from build123d import *

# Parameters (mm, degrees)
SKETCH_1_R      = 33.5
SKETCH_1_R_2    = 23.5
EXTRUDE_1_DEPTH = 25
SKETCH_2_R      = 10
EXTRUDE_2_DEPTH = 2
SKETCH_3_R      = 5
SKETCH_3_R_2    = 2.5
EXTRUDE_3_DEPTH = 20


with BuildPart() as part:
    # 草圖1 → 填料-伸長1 (new body)
    with BuildSketch(Plane.XY):
        Circle(SKETCH_1_R)
        Circle(SKETCH_1_R_2, mode=Mode.SUBTRACT)
    extrude(amount=EXTRUDE_1_DEPTH)

    # 草圖2 → 填料-伸長2 (add)
    with BuildSketch(Plane(origin=(0, 0, 0), x_dir=(-1, 0, 0), z_dir=(0, 0, -1))):
        with BuildLine():
            ThreePointArc((-5, 8.660254038), (-2.588190451, 9.659258263), (0, 10))
            Line((0, 10), (0, 23.5))
            ThreePointArc((0, 23.5), (-1.251777149, 23.46663704), (-2.5, 23.366642891))
            Line((-2.5, 23.366642891), (-5, 8.660254038))
        make_face()
        with BuildLine():
            Line((0, 23.5), (0, 10))
            ThreePointArc((0, 10), (2.588190451, 9.659258263), (5, 8.660254038))
            Line((5, 8.660254038), (2.5, 23.366642891))
            ThreePointArc((2.5, 23.366642891), (1.251777149, 23.46663704), (0, 23.5))
        make_face()
        Circle(SKETCH_2_R)
        with BuildLine():
            ThreePointArc((-9.781476007, -2.079116908), (-9.510565163, 3.090169944), (-6.691306064, 7.431448255))
            Line((-6.691306064, 7.431448255), (-21.4504555, 9.598331046))
            ThreePointArc((-21.4504555, 9.598331046), (-22.349828133, 7.261899368), (-22.995540471, 4.843048464))
            Line((-22.995540471, 4.843048464), (-9.781476007, -2.079116908))
        make_face()
        with BuildLine():
            ThreePointArc((-1.045284633, -9.945218954), (-5.877852523, -8.090169944), (-9.135454576, -4.067366431))
            Line((-9.135454576, -4.067366431), (-15.757110573, -17.43454807))
            ThreePointArc((-15.757110573, -17.43454807), (-13.812953429, -19.011899368), (-11.712025601, -20.373474331))
            Line((-11.712025601, -20.373474331), (-1.045284633, -9.945218954))
        make_face()
        with BuildLine():
            Line((15.757110573, -17.43454807), (9.135454576, -4.067366431))
            ThreePointArc((9.135454576, -4.067366431), (5.877852523, -8.090169944), (1.045284633, -9.945218954))
            Line((1.045284633, -9.945218954), (11.712025601, -20.373474331))
            ThreePointArc((11.712025601, -20.373474331), (13.812953429, -19.011899368), (15.757110573, -17.43454807))
        make_face()
        with BuildLine():
            Line((21.4504555, 9.598331046), (6.691306064, 7.431448255))
            ThreePointArc((6.691306064, 7.431448255), (9.135454576, 4.067366431), (10, 0))
            ThreePointArc((10, 0), (9.945218954, -1.045284633), (9.781476007, -2.079116908))
            Line((9.781476007, -2.079116908), (22.995540471, 4.843048464))
            ThreePointArc((22.995540471, 4.843048464), (22.349828133, 7.261899368), (21.4504555, 9.598331046))
        make_face()
    extrude(amount=-EXTRUDE_2_DEPTH)

    # 草圖3 → 填料-伸長3 (add)
    with BuildSketch(Plane.XY.offset(2)):
        with Locations(Location((0, 0, 0), (0, 0, 180))):
            Circle(SKETCH_3_R)
        Circle(SKETCH_3_R_2, mode=Mode.SUBTRACT)
    extrude(amount=EXTRUDE_3_DEPTH)


solid = part.part
Work out the finished part from the listing and answer in its coordinate system (mm). A direction names the side the tool comes from. Give positions to 0.01 mm unless a question says otherwise; leave off trailing zeros. Loops run counter-clockwise (first coordinate to the right, second up) from the corner with the lowest first, then second, coordinate; pieces in that order, holes last. Notation, with made-up numbers: (50, 29.5) - (96, 29.5) arc R15 ccw to (96, 56.5) - close; hole circle Ø6 at (12, 60.25). An arc over 180 degrees is marked (long way). Answer in a Markdown table with one row per item.
(1) Flat-ended cylindrical pins translate along their axes: pin 1 Ø4 at (y, z) = (-8, 22) entering from -X; pin 2 Ø3 at (x, y) = (0, 0) entering from -Z; pin 3 Ø3 at (y, z) = (-23, 5) entering from -X; pin 4 Ø3 at (x, y) = (-1.5, -1.5) entering from +Z. Find the tip coordinate at first contact, or state that the pin passes through.
Results list:
| item | result |
|---|---|
| pin 1 | stops at x = -32.96 |
| pin 2 | stops at z = 0 |
| pin 3 | stops at x = -25.69 |
| pin 4 | stops at z = 22 |
(2) Section D-D (x = -17.5) is taken. Give the vertices of the cut face in (y, z).
Results list:
| item | result |
|---|---|
| outline | (-28.57, 0) - (-15.68, 0) - (-15.68, 25) - (-28.57, 25) - close; (1.96, 0) - (9.02, 0) - (9.02, 2) - (1.96, 2) - close; (15.68, 0) - (28.57, 0) - (28.57, 25) - (15.68, 25) - close |
(3) Section B-B (z = 18) is taken. Give the vertices of the cut face in (x, y).
Results list:
| item | result |
|---|---|
| outline | circle Ø67 at (0, 0); circle Ø10 at (0, 0); hole circle Ø47 at (0, 0); hole circle Ø5 at (0, 0) |
(4) For a pull along X with two mould halves and no side action, classify faces 1 (the face through (-23, -7, 25)), 2 (the face through (6, 8, 1)), 3 (the face through (-7.262, -32.703, 12.325)) as pulls with the +X half, pulls with the -X half, needs draft (parallel to the pull), parting line crosses it, or undercut.
Results list:
| item | result |
|---|---|
| face 1 | needs draft |
| face 2 | undercut |
| face 3 | parting line crosses it |
(5) A tool of negligible diameter and unlimited length cuts with its end or side. For faces 4 (the face through (-2, 2, 22)), 5 (the face through (0, 0, 0)), 6 (the face through (9.515, -3.076, 0.986)), from which of +Z, -Z, +X, -X, +Y, -Y can it reach the whole face along a straight path? Write none if from no direction.
Results list:
| item | result |
|---|---|
| face 4 | +Z |
| face 5 | -Z, +X, -X, +Y, -Y |
| face 6 | +Z, -Z |
(6) Consider L1, parallel to Y at x = 0, z = 8.5; L2, parallel to X at y = -3.5, z = 16.25; L3, parallel to Y at x = 18.5, z = 21.5. Determine where each line is inside the solid, lowest interval first. Write a range as [from, to].
Results list:
| item | result |
|---|---|
| L1 | y = [-33.5, -23.5], [-5, -2.5], [2.5, 5], [23.5, 33.5] |
| L2 | x = [-33.32, -23.24], [-3.57, 3.57], [23.24, 33.32] |
| L3 | y = [-27.93, -14.49], [14.49, 27.93] |
(7) Section C-C (y = 20) is taken. Give the vertices of the cut face in (x, z).
Results list:
| item | result |
|---|---|
| outline | (-26.87, 0) - (-12.34, 0) - (-12.34, 25) - (-26.87, 25) - close; (-3.07, 0) - (3.07, 0) - (3.07, 2) - (-3.07, 2) - close; (12.34, 0) - (26.87, 0) - (26.87, 25) - (12.34, 25) - close |
(8) Section A-A (x = 0) is taken. Give the vertices of the cut face in (y, z), and give its area (3 significant figures).
Results list:
| item | result |
|---|---|
| outline | (-33.5, 0) - (-23.5, 0) - (-23.5, 25) - (-33.5, 25) - close; (-10, 0) - (33.5, 0) - (33.5, 25) - (23.5, 25) - (23.5, 2) - (5, 2) - (5, 22) - (2.5, 22) - (2.5, 2) - (-2.5, 2) - (-2.5, 22) - (-5, 22) - (-5, 2) - (-10, 2) - close |
| area | 667 mm² |
